Can you work these out from the model? Positions are in its coordinate system, mm. A direction names the side the tool comes from. Round coordinates to 2 decimals unless told otherwise and drop trailing zeros. Loops run counter-clockwise (first coordinate to the right, second up) from the corner with the lowest first, then second, coordinate; pieces in that order, holes last. Notation, with made-up numbers: (27.5, -15) -> (48.5, -15) arc R21 cw to (48.5, 0) -> close; hole circle Ø10 at (79, 41.5). An arc over 180 degrees is marked (long way). Write item = value, one per line.
Autodesk Inventor part; units mm, degrees
ref_plane "YZ Plane" through (0, 0, 0) normal (1, 0, 0) x (0, 1, 0)
ref_plane "XZ Plane" through (0, 0, 0) normal (0, 1, 0) x (-1, 0, 0)
ref_plane "XY Plane" through (0, 0, 0) normal (0, 0, 1) x (1, 0, 0)
sketch "Esquisse1" plane through (0, 0, 0) normal (0, 1, 0) x (-1, 0, 0)
  line L0 (-55, 100) -> (55, 100)
  line L1 (55, 100) -> (55, -100)
  line L2 (55, -100) -> (-55, -100)
  line L3 (-55, -100) -> (-55, 100)
  line L4 (-55, 100) -> (55, -100) construction
  line L5 (55, 100) -> (-55, -100) construction
  point P0 (0, 0)
  dimension "d0" = 110
  dimension "d1" = 200
extrude "Extrusion1" add sketch "Esquisse1" along normal blind 5
sketch "Esquisse4" plane through (0, 5, 0) normal (0, 1, 0) x (1, 0, 0)
  line L0 (0, 0) -> (0, 60)
  dimension "d22" = 60
hole "Perçage3" at (0, 5, -60) direction (0, -1, 0) diameter 7.6468 end through all
sketch "Esquisse5" plane through (0, 5, 0) normal (0, 1, 0) x (1, 0, 0)
  line L0 (-55, -100) -> (55, -100)
  line L1 (0, -100) -> (-27.5, -100)
  line L2 (-27.5, -100) -> (-27.5, -70)
  line L3 (-27.5, -70) -> (-37.5, -70)
  line L4 (-27.5, -70) -> (-7.5, -70)
  line L5 (-37.5, -70) -> (-37.5, -55)
  line L6 (-7.5, -55) -> (-7.5, -70)
  point P0 (0, 0)
  dimension "d30" = 27.5
  dimension "d31" = 30
  dimension "d32" = 10
  dimension "d33" = 20
  dimension "d34" = 15
hole "Perçage4" at (-7.5, 5, 70) at (-37.5, 5, 70) at (-37.5, 5, 55) at (-7.5, 5, 55) direction (0, -1, 0) diameter 2.459 end through all
sketch "Esquisse6" plane through (-55, 0, 100) normal (0, 0, 1) x (1, 0, 0)
  line L0 (0, 0) -> (110, 0)
  line L1 (110, 0) -> (110, 5)
  line L2 (0, 5) -> (110, 5)
  line L3 (0, 0) -> (0, 5)
  point P0 (55, 0)
extrude "Extrusion2" add sketch "Esquisse6" along normal blind 40
sketch "Esquisse7" plane through (0, 5, 0) normal (0, 1, 0) x (1, 0, 0)
  circle A0 centre (0, 60) radius 3.8234
  circle A1 centre (0, 60) radius 3.5
  circle A2 centre (0, 60) radius 4.75
  point P0 (0, 0)
  dimension "d47" = 7
  dimension "d48" = 9.5
extrude "Extrusion3" add sketch "Esquisse7" along normal blind 1 contours A0 | A2
sketch "Esquisse8" plane through (0, 5, 0) normal (0, 1, 0) x (1, 0, 0)
  line L0 (-55, 100) -> (-55, -140)
  line L1 (55, 100) -> (55, -140)
  line L2 (-55, -140) -> (55, -140)
  line L3 (55, -140) -> (55, 30)
  line L4 (55, 30) -> (-55, 30)
  line L5 (-55, 30) -> (-55, -140)
  point P0 (0, 0)
  dimension "d51" = 170
extrude "Extrusion4" cut sketch "Esquisse8" against normal blind 10
sketch "Esquisse9" plane through (0, 5, 0) normal (0, 1, 0) x (1, 0, 0)
  line L0 (-55, 30) -> (55, 30)
  line L1 (-55, 30) -> (-55, 32.5)
  line L2 (-55, 100) -> (-55, 30)
  line L3 (-55, 32.5) -> (-52.5, 32.5)
  line L4 (55, 30) -> (55, 32.5)
  line L5 (55, 100) -> (55, 30)
  line L6 (55, 32.5) -> (52.5, 32.5)
  point P0 (0, 0)
  dimension "d54" = 2.5
  dimension "d55" = 2.5
  dimension "d56" = 2.5
  dimension "d57" = 2.5
hole "Perçage5" at (-52.5, 5, -32.5) at (52.5, 5, -32.5) direction (0, -1, 0) diameter 2.459 end through all
sketch "Esquisse10" plane through (0, 5, 0) normal (0, 1, 0) x (1, 0, 0)
  line L0 (55, 100) -> (-55, 100)
  line L1 (55, 100) -> (55, 30)
  line L2 (-55, 100) -> (55, 100)
  line L3 (55, 100) -> (55, 95)
  line L4 (55, 95) -> (-55, 95)
  line L5 (-55, 95) -> (-55, 100)
  point P0 (0, 0)
  dimension "d65" = 5
extrude "Extrusion5" cut sketch "Esquisse10" against normal blind 10
sketch "Esquisse11" plane through (0, 5, 0) normal (0, 1, 0) x (1, 0, 0)
  line L0 (-55, 95) -> (-52.5, 95)
  line L1 (55, 95) -> (-55, 95)
  line L2 (-52.5, 95) -> (-52.5, 92.5)
  line L3 (55, 95) -> (55, 30)
  line L4 (55, 95) -> (52.5, 95)
  line L5 (52.5, 95) -> (52.5, 92.5)
  point P0 (0, 0)
  dimension "d68" = 2.5
  dimension "d69" = 2.5
  dimension "d70" = 2.5
hole "Perçage6" at (-52.5, 5, -92.5) at (52.5, 5, -92.5) direction (0, -1, 0) diameter 2.459 end through all
sketch "Esquisse12" plane through (55, 5, -95) normal (0, 0, -1) x (-1, 0, 0)
  line L0 (0, -5) -> (0, 0)
  line L1 (0, 0) -> (5.1, 0)
  line L2 (110, 0) -> (0, 0)
  line L3 (5.1, 0) -> (5.1, -1.1)
  line L4 (5.1, -1.1) -> (24.9, -1.1)
  line L5 (24.9, -1.1) -> (24.9, -3.9)
  line L6 (24.9, -3.9) -> (5.1, -3.9)
  line L7 (5.1, -3.9) -> (5.1, -1.1)
  line L8 (110, -5) -> (110, 0)
  line L9 (110, 0) -> (104.9, 0)
  line L10 (104.9, 0) -> (104.9, -1.1)
  line L11 (104.9, -1.1) -> (85.1, -1.1)
  line L12 (85.1, -1.1) -> (85.1, -3.9)
  line L13 (85.1, -3.9) -> (104.9, -3.9)
  line L14 (104.9, -3.9) -> (104.9, -1.1)
  line L15 (110, -5) -> (0, -5)
  point P0 (55, -5)
  dimension "d78" = 5.1
  dimension "d79" = 1.1
  dimension "d80" = 19.8
  dimension "d81" = 2.8
  dimension "d82" = 5.1
  dimension "d83" = 19.8
  dimension "d86" = 1.1
  dimension "d87" = 1.1
extrude "Extrusion6" add sketch "Esquisse12" along normal blind 7 contours L14 L13 L12 L11 | L4 L5 L6 L7
sketch "Esquisse13" plane through (0, 6, -60) normal (0, 1, 0) x (1, 0, 0)
  circle A0 centre (0, 0) radius 3.95
  circle A1 centre (0, 0) radius 3.5
  point P0 (0, -60)
  dimension "d88" = 7.9
  dimension "d89" = 7
extrude "Extrusion7" add sketch "Esquisse13" along normal blind 6
properties part number "chassis_haut"
1. We'd pull the mould along X, two halves only. Please class faces 4 (the flat face through (55, 2, -63)), 5 (the cylindrical face through (1.615, 8.451, -63.105)), 6 (the flat face through (-1, 0, -70)): released by +X, released by -X, zero draft, split by the parting line, or undercut.
Entries:
face_4 = released by +X
face_5 = undercut
face_6 = zero draft
2. Suppose I cut it at B-B, the plane x = 0. List the corners of the cut face in (y, z) for me, and give its area (3 significant figures).
Entries:
outline = (0, -95) -> (5, -95) -> (5, -64.75) -> (6, -64.75) -> (6, -63.95) -> (12, -63.95) -> (12, -63.5) -> (5, -63.5) -> (5, -63.82) -> (0, -63.82) -> close; (0, -56.18) -> (5, -56.18) -> (5, -56.5) -> (12, -56.5) -> (12, -56.05) -> (6, -56.05) -> (6, -55.25) -> (5, -55.25) -> (5, -30) -> (0, -30) -> close
area = 295 mm²
3. I need wall thicknesses on line 1 (X direction, y = 1.3, z = -32.5); line 2 (Z direction, x = -52.5, y = 3.65); line 3 (Z direction, x = 0, y = 2.65). Which ranges of each line are inside material? Lowest first, please. Write a range as [from, to].
Entries:
line_1 = [-55, -53.73], [-51.27, 51.27], [53.73, 55]
line_2 = [-95, -93.73], [-91.27, -33.73], [-31.27, -30]
line_3 = [-95, -63.82], [-56.18, -30]
4. I'm going to push flat-ended pins straight in: pin 1 (6.5 mm diameter, centred on x = 0, z = -60, fed in from -Y); pin 2 (3 mm diameter, centred on y = 2, z = -98.5, fed in from -X); pin 3 (6 mm diameter, centred on x = -29.5, z = -41, fed in from +Y); pin 4 (2 mm diameter, centred on x = 42.5, z = -98.5, fed in from -Y). Where does each tip first touch, or does it pass through?
Entries:
pin_1 = through
pin_2 = -49.9
pin_3 = 5
pin_4 = 1.1
5. Suppose I cut it at D-D, the plane x = -52.5. List the corners of the cut face in (y, z) for me.
Entries:
outline = (0, -95) -> (5, -95) -> (5, -93.73) -> (0, -93.73) -> close; (0, -91.27) -> (5, -91.27) -> (5, -33.73) -> (0, -33.73) -> close; (0, -31.27) -> (5, -31.27) -> (5, -30) -> (0, -30) -> close
6. Suppose I cut it at A-A, the plane z = -60. List the corners of the cut face in (x, y) for me, and give its area (3 significant figures).
Entries:
outline = (-55, 0) -> (-3.82, 0) -> (-3.82, 5) -> (-3.5, 5) -> (-3.5, 12) -> (-3.95, 12) -> (-3.95, 6) -> (-4.75, 6) -> (-4.75, 5) -> (-55, 5) -> close; (3.5, 5) -> (3.82, 5) -> (3.82, 0) -> (55, 0) -> (55, 5) -> (4.75, 5) -> (4.75, 6) -> (3.95, 6) -> (3.95, 12) -> (3.5, 12) -> close
area = 520 mm²
7. Suppose I cut it at C-C, the plane z = -32.5. List the corners of the cut face in (x, y) for me, and give its area (3 significant figures).
Entries:
outline = (-55, 0) -> (-53.73, 0) -> (-53.73, 5) -> (-55, 5) -> close; (-51.27, 0) -> (51.27, 0) -> (51.27, 5) -> (-51.27, 5) -> close; (53.73, 0) -> (55, 0) -> (55, 5) -> (53.73, 5) -> close
area = 525 mm²
8. For faces 1 (the flat face through (-40, 1.1, -98)), 2 (the flat face through (-30.1, 3, -98)), 3 (the flat face through (49.9, 2, -98)), which set-ups out of +Z, -Z, +X, -X, +Y, -Y let a thin tool reach every point of the face, with its end or its side?
Entries:
face_1 = -Z, +X, -X, -Y
face_2 = -Z, +Y, -Y
face_3 = -Z, +X, +Y, -Y
